Can you work these out from the model? Positions are in its coordinate system, mm. A direction names the side the tool comes from. Give positions to 0.01 mm unless a question says otherwise; leave off trailing zeros. Write each loop counter-clockwise with the first axis right and the second up, starting at its lowest first coordinate (ties: lowest second). Pieces come first, ordered by that corner, then holes. Notation, with made-up numbers: (25.5, -27) -> (69.5, -27) arc R18 cw to (69.5, -6) -> close; hole circle Ø6 at (68.25, -10). An arc over 180 degrees is marked (long way). One line per item, written item: value.
Autodesk Inventor part; units mm, degrees
ref_plane "YZ Plane" through (0, 0, 0) normal (1, 0, 0) x (0, 1, 0)
ref_plane "XZ Plane" through (0, 0, 0) normal (0, 1, 0) x (-1, 0, 0)
ref_plane "XY Plane" through (0, 0, 0) normal (0, 0, 1) x (1, 0, 0)
sketch "Sketch1" plane through (0, 0, 0) normal (0, 1, 0) x (-1, 0, 0)
  line L0 (59.6914, -40.823) -> (-60.3086, -40.823)
  line L1 (-65.3086, -35.823) -> (-65.3086, 34.177)
  line L2 (-60.3086, 39.177) -> (59.6914, 39.177)
  line L3 (64.6914, 34.177) -> (64.6914, -35.823)
  arc A0 (59.6914, -40.823) -> (64.6914, -35.823) centre (59.6914, -35.823) ccw
  arc A1 (-65.3086, -35.823) -> (-60.3086, -40.823) centre (-60.3086, -35.823) ccw
  arc A2 (64.6914, 34.177) -> (59.6914, 39.177) centre (59.6914, 34.177) ccw
  arc A3 (-60.3086, 39.177) -> (-65.3086, 34.177) centre (-60.3086, 34.177) ccw
  point P0 (0, 0)
  point P1 (64.6914, -40.823)
  point P2 (-65.3086, 39.177)
  point P3 (64.6914, 39.177)
  dimension "d0" = 80
  dimension "d1" = 130
  dimension "d2" = 5
  dimension "d3" = 5
  dimension "d4" = 5
  dimension "d5" = 5
extrude "Extrusion1" add sketch "Sketch1" along normal blind 2
sketch "Sketch2" plane through (0, 2, 0) normal (0, 1, 0) x (1, 0, 0)
  line L0 (-64.6914, 35.823) -> (-64.6914, -34.177)
  line L1 (-64.6914, 35.823) -> (-64.6914, -34.177)
  arc A0 (-64.6914, -34.177) -> (-59.6914, -39.177) centre (-59.6914, -34.177) ccw
  arc A1 (-64.6914, -34.177) -> (-59.6914, -39.177) centre (-59.6914, -34.177) ccw
  arc A2 (-59.6914, 40.823) -> (-64.6914, 35.823) centre (-59.6914, 35.823) ccw
  arc A3 (65.3086, 35.823) -> (60.3086, 40.823) centre (60.3086, 35.823) ccw
  arc A4 (65.3086, 35.823) -> (60.3086, 40.823) centre (60.3086, 35.823) ccw
  line L2 (-62.1914, 35.823) -> (-62.1914, -34.177)
  line L3 (65.3086, -34.177) -> (65.3086, 35.823)
  line L4 (65.3086, 35.823) -> (65.3086, -34.177)
  arc A5 (60.3086, -39.177) -> (65.3086, -34.177) centre (60.3086, -34.177) ccw
  line L5 (-59.6914, -39.177) -> (60.3086, -39.177)
  line L6 (60.3086, -39.177) -> (-59.6914, -39.177)
  line L7 (60.3086, 40.823) -> (-59.6914, 40.823)
  line L8 (-59.6914, 40.823) -> (60.3086, 40.823)
  line L9 (62.8086, 35.823) -> (62.8086, -34.177)
  line L10 (60.3086, -36.677) -> (-59.6914, -36.677)
  line L11 (-59.6914, 38.323) -> (60.3086, 38.323)
  arc A6 (-59.6914, 38.323) -> (-62.1914, 35.823) centre (-59.6914, 35.823) ccw
  arc A7 (62.8086, 35.823) -> (60.3086, 38.323) centre (60.3086, 35.823) ccw
  arc A8 (60.3086, -36.677) -> (62.8086, -34.177) centre (60.3086, -34.177) ccw
  arc A9 (-62.1914, -34.177) -> (-59.6914, -36.677) centre (-59.6914, -34.177) ccw
  arc A10 (-59.6914, 39.323) -> (-63.1914, 35.823) centre (-59.6914, 35.823) ccw
  arc A11 (63.8086, 35.823) -> (60.3086, 39.323) centre (60.3086, 35.823) ccw
  arc A12 (60.3086, -37.677) -> (63.8086, -34.177) centre (60.3086, -34.177) ccw
  arc A13 (-63.1914, -34.177) -> (-59.6914, -37.677) centre (-59.6914, -34.177) ccw
  line L12 (-63.1914, 35.823) -> (-63.1914, -34.177)
  line L13 (-59.6914, -37.677) -> (60.3086, -37.677)
  line L14 (63.8086, -34.177) -> (63.8086, 35.823)
  line L15 (60.3086, 39.323) -> (-59.6914, 39.323)
  line L16 (-59.6914, 32.323) -> (-62.1914, 32.323)
  line L17 (-56.1914, 35.823) -> (-56.1914, 38.323)
  arc A14 (-59.6914, 32.323) -> (-56.1914, 35.823) centre (-59.6914, 35.823) ccw
  line L18 (0.3086, 40.823) -> (0.3086, 33.323)
  line L19 (65.3086, 0.823) -> (44.6486, 0.823)
  line L20 (60.3086, 32.323) -> (62.8086, 32.323)
  line L21 (56.8086, 35.823) -> (56.8086, 38.323)
  arc A15 (56.8086, 35.823) -> (60.3086, 32.323) centre (60.3086, 35.823) ccw
  line L22 (-59.6914, -30.677) -> (-62.1914, -30.677)
  line L23 (-56.1914, -34.177) -> (-56.1914, -36.677)
  arc A16 (-56.1914, -34.177) -> (-59.6914, -30.677) centre (-59.6914, -34.177) ccw
  line L24 (56.8086, -34.177) -> (56.8086, -36.677)
  arc A17 (60.3086, -30.677) -> (56.8086, -34.177) centre (60.3086, -34.177) ccw
  line L25 (60.3086, -30.677) -> (62.8086, -30.677)
  point P0 (0, 0)
  point P1 (60.3086, -34.2192)
  point P2 (65.3086, -34.2192)
  point P3 (59.6599, -39.177)
  point P4 (56.8086, 38.323)
  point P5 (62.8086, -30.677)
  point P6 (56.8086, -36.677)
  point P7 (-56.1914, -36.677)
  point P8 (-62.1914, -30.677)
  dimension "d51" = 5
  dimension "d8" = 2.5
  dimension "d9" = 2.5
  dimension "d10" = 2.5
  dimension "d11" = 2.5
  dimension "d12" = 7
  dimension "d13" = 7
  dimension "d14" = 7
  dimension "d15" = 7
  dimension "d34" = 3.5
  dimension "d50" = 2.5
  dimension "d52" = 5
  dimension "d53" = 2.5
extrude "Extrusion2" add sketch "Sketch2" along normal blind 5 contours A2 L7 L18 L15 A10 L12 A13 L13 A12 L14 L19 L3 A5 L5 A0 L0 | L7 A3 L3 L19 L14 A11 L15 L18 | L17 A14 L16 L2 A6 L11 | L11 A7 L9 L20 A15 L21 | L9 A8 L10 L24 A17 L25 | L22 A16 L23 L10 A9 L2
extrude "Extrusion3" add sketch "Sketch2" along normal blind 6 contours L18 L11 A6 L2 A9 L10 A8 L9 L19 L14 A12 L13 A13 L12 A10 L15 | L15 A11 L14 L19 L9 A7 L11 L18 | L17 A14 L16 L2 A6 L11 | L11 A7 L9 L20 A15 L21 | L9 A8 L10 L24 A17 L25 | L22 A16 L23 L10 A9 L2
sketch "Sketch3" plane through (0, 0, 0) normal (0, -1, 0) x (1, 0, 0)
  circle A0 centre (60.3086, 34.177) radius 3
  line L0 (-59.6914, 39.177) -> (60.3086, 39.177)
  line L1 (65.3086, 34.177) -> (65.3086, -35.823)
  line L2 (65.3086, 24.0261) -> (65.3086, 17.2129)
  line L3 (38.477, 39.177) -> (29.3328, 39.177)
  line L4 (-59.6914, 39.177) -> (60.3086, 39.177)
  circle A1 centre (60.3086, -35.823) radius 3
  circle A2 centre (-59.6914, 34.177) radius 3
  circle A3 centre (-59.6914, -35.823) radius 3
  line L5 (-64.6914, -35.823) -> (-64.6914, 34.177)
  line L6 (60.3086, -40.823) -> (-59.6914, -40.823)
  point P0 (0, 0)
  point P1 (33.602, 39.1426)
  point P2 (55.3086, 34.177)
  point P3 (65.3086, -35.823)
  dimension "d20" = 6
  dimension "d21" = 5
  dimension "d26" = 70
  dimension "d29" = 120
  dimension "d54" = 130
  dimension "d55" = 80
  dimension "d56" = 5
extrude "Extrusion4" cut sketch "Sketch3" against normal blind 3
sketch "Sketch4" plane through (60.3086, 3, -35.823) normal (0, -1, 0) x (1, 0, 0)
  circle A0 centre (0, 0) radius 3
  point P0 (-60.3086, 35.823)
hole "Hole1" at (60.3086, 3, -35.823) direction (0, 1, 0) diameter 3.5 end through all
pattern_linear "Rectangular Pattern1" count 2 spacing 120 along (-1, 0, 0) count 2 spacing 70 along (0, 0, 1) of "Hole1"
chamfer "Chamfer1" distance 1 angle 45 8 edges at (0.3086, 0, 39.177) (63.8442, 0, 37.7125) (65.3086, 0, -0.823) (63.8442, 0, -39.3586) (0.3086, 0, -40.823) (-63.2269, 0, -39.3586) (-64.6914, 0, -0.823) (-63.2269, 0, 37.7125)
sketch "Sketch9" plane through (0, 0, 0) normal (0, -1, 0) x (1, 0, 0)
  line L0 (-8.8254, 34.5739) -> (9.2353, 34.5739) construction
  line L1 (9.2353, 34.5739) -> (9.2353, 29.7737) construction
  line L2 (9.2353, 29.7737) -> (-8.8254, 29.7737) construction
  line L3 (-8.8254, 29.7737) -> (-8.8254, 34.5739) construction
  point P0 (0, 0)
sketch "Sketch10" plane through (0, 2, 0) normal (0, 1, 0) x (1, 0, 0)
  line L0 (46.8086, -34.677) -> (-3.1914, -34.677)
  line L1 (-3.1914, -34.677) -> (-3.1914, -32.677)
  line L2 (-3.1914, -32.677) -> (46.8086, -32.677)
  line L3 (46.8086, -32.677) -> (46.8086, -34.677)
  line L4 (56.8086, -34.177) -> (56.8086, -36.677)
  line L5 (56.8086, -36.677) -> (-56.1914, -36.677)
  line L6 (-46.1914, 36.323) -> (3.8086, 36.323)
  line L7 (3.8086, 36.323) -> (3.8086, 34.323)
  line L8 (3.8086, 34.323) -> (-46.1914, 34.323)
  line L9 (-46.1914, 34.323) -> (-46.1914, 36.323)
  line L10 (-56.1914, 38.323) -> (56.8086, 38.323)
  line L11 (-56.1914, 35.823) -> (-56.1914, 38.323)
  point P0 (0, 0)
  point P1 (56.8086, -35.427)
  point P2 (46.8086, -33.677)
  point P3 (-3.1914, -36.677)
  point P4 (-46.1914, 35.323)
  point P5 (-56.1914, 37.073)
  dimension "d97" = 50
  dimension "d98" = 2
  dimension "d99" = 10
  dimension "d100" = 2
  dimension "d110" = 50
  dimension "d111" = 2
  dimension "d112" = 2
  dimension "d113" = 10
extrude "Extrusion7" add sketch "Sketch10" along normal blind 5
chamfer "Chamfer2" distance 1 angle 60 1 edges at (21.8086, 7, 34.677) measured on face at (13.4753, 7, 33.3436)
chamfer "Chamfer4" distance 1 angle 60 1 edges at (-21.1914, 7, -36.323) measured on face at (-29.5247, 7, -35.6564)
sketch "Sketch11" plane through (0, 0, 0) normal (0, -1, 0) x (1, 0, 0)
  line L0 (-56.6914, 5.177) -> (-16.6914, 5.177)
  line L1 (-16.6914, 5.177) -> (-16.6914, -20.823)
  line L2 (-16.6914, -20.823) -> (-56.6914, -20.823)
  line L3 (-56.6914, -20.823) -> (-56.6914, 5.177)
  line L4 (-64.6914, 34.177) -> (-64.6914, -35.823)
  line L5 (-59.6914, -40.823) -> (60.3086, -40.823)
  point P0 (0, 0)
  dimension "d117" = 40
  dimension "d118" = 26
  dimension "d119" = 8
  dimension "d120" = 20
extrude "Extrusion8" cut sketch "Sketch11" against normal blind 10
sketch "Sketch12" plane through (0, 2, 0) normal (0, 1, 0) x (1, 0, 0)
  line L0 (-57.6914, 28.823) -> (-15.6914, 28.823)
  line L1 (-15.6914, 28.823) -> (-15.6914, -13.177)
  line L2 (-15.6914, -13.177) -> (-57.6914, -13.177)
  line L3 (-57.6914, -13.177) -> (-57.6914, 28.823)
  line L4 (-16.6914, -5.177) -> (-56.6914, -5.177)
  line L5 (-16.6914, 20.823) -> (-16.6914, -5.177)
  circle A0 centre (-54.1914, 25.323) radius 1.75
  circle A1 centre (-19.1914, 25.323) radius 1.75
  circle A2 centre (-54.1914, -9.677) radius 1.75
  circle A3 centre (-19.1914, -9.677) radius 1.75
  point P0 (0, 0)
  dimension "d127" = 42
  dimension "d128" = 42
  dimension "d129" = 8
  dimension "d130" = 1
  dimension "d131" = 3.5
  dimension "d132" = 3.5
  dimension "d133" = 3.5
  dimension "d136" = 35
  dimension "d139" = 35
extrude "Extrusion9" cut sketch "Sketch12" against normal blind 10 contours A0 | A1 | A2 | A3
sketch "Sketch13" plane through (0, 2, 0) normal (0, 1, 0) x (1, 0, 0)
  line L0 (-57.6914, -6.177) -> (-15.6914, -6.177)
  line L1 (-15.6914, -6.177) -> (-15.6914, 21.823)
  line L2 (-15.6914, 21.823) -> (-57.6914, 21.823)
  line L3 (-57.6914, 21.823) -> (-57.6914, -6.177)
  line L4 (-56.6914, 20.823) -> (-16.6914, 20.823)
  line L5 (-56.6914, -5.177) -> (-16.6914, -5.177)
  line L6 (-16.6914, -5.177) -> (-16.6914, 20.823)
  line L7 (-16.6914, 20.823) -> (-56.6914, 20.823)
  line L8 (-56.6914, 20.823) -> (-56.6914, -5.177)
  point P0 (0, 0)
  dimension "d144" = 1
  dimension "d145" = 1
  dimension "d146" = 1
  dimension "d147" = 1
extrude "Extrusion10" add sketch "Sketch13" along normal blind 3.8
equation "\"d3\" = d2"
equation "\"d4\" = d2"
equation "\"d5\" = d2"
equation "\"d9\" = d8"
equation "\"d10\" = d8"
equation "\"d11\" = d8"
equation "\"d52\" = d51"
equation "\"d53\" = d50"
properties part number "housing_top"
1) If we section it at D-D (x = 38): Write out the boundary of the cut face in (y, z), and give its area (3 significant figures).
Answer list:
outline: (0, -39.82) -> (1, -40.82) -> (7, -40.82) -> (7, -39.32) -> (8, -39.32) -> (8, -38.32) -> (2, -38.32) -> (2, 32.68) -> (7, 32.68) -> (7, 33.68) -> (5.27, 34.68) -> (2, 34.68) -> (2, 36.68) -> (8, 36.68) -> (8, 37.68) -> (7, 37.68) -> (7, 39.18) -> (1, 39.18) -> (0, 38.18) -> close
area: 195 mm^2
2) Will these pins go through, and if not, where does the flat tip stop? pin 1 (22.5 mm diameter, centred on x = -1.5, z = -7, fed in from +Y); pin 2 (14 mm diameter, centred on x = -32, z = -12.5, fed in from +Y); pin 3 (0.8 mm diameter, centred on y = 7.5, z = -10, fed in from +X); pin 4 (1.1 mm diameter, centred on x = -25, z = -35, fed in from +Y).
Answer list:
pin 1: stops at y = 2
pin 2: passes through
pin 3: stops at x = 63.81
pin 4: stops at y = 7
3) I need wall thicknesses on L1, parallel to Z at x = 41.5, y = 4; L2, parallel to Z at x = 60.5, y = 5; L3, parallel to X at y = 4.5, z = -13. Which ranges of each line are inside material? Lowest first, please.
Answer list:
L1: z = -40.82 to -38.32, 32.68 to 34.68, 36.68 to 39.18
L2: z = -40.82 to -37.56, -34.08 to -32.32, 30.68 to 32.44, 35.92 to 39.17
L3: x = -64.69 to -62.19, -57.69 to -56.69, -16.69 to -15.69, 62.81 to 65.31
4) If we section it at C-C (x = -37): Write out the boundary of the cut face in (y, z).
Answer list:
outline: (0, -39.82) -> (1, -40.82) -> (7, -40.82) -> (7, -39.32) -> (8, -39.32) -> (8, -38.32) -> (2, -38.32) -> (2, -36.32) -> (5.27, -36.32) -> (7, -35.32) -> (7, -34.32) -> (2, -34.32) -> (2, -21.82) -> (5.8, -21.82) -> (5.8, -20.82) -> (0, -20.82) -> close; (0, 5.18) -> (5.8, 5.18) -> (5.8, 6.18) -> (2, 6.18) -> (2, 36.68) -> (8, 36.68) -> (8, 37.68) -> (7, 37.68) -> (7, 39.18) -> (1, 39.18) -> (0, 38.18) -> close
5) If we section it at B-B (z = -7): Write out the boundary of the cut face in (x, y), and give its area (3 significant figures).
Answer list:
outline: (-64.69, 1) -> (-63.69, 0) -> (-56.69, 0) -> (-56.69, 5.8) -> (-57.69, 5.8) -> (-57.69, 2) -> (-62.19, 2) -> (-62.19, 8) -> (-63.19, 8) -> (-63.19, 7) -> (-64.69, 7) -> close; (-16.69, 0) -> (64.31, 0) -> (65.31, 1) -> (65.31, 7) -> (63.81, 7) -> (63.81, 8) -> (62.81, 8) -> (62.81, 2) -> (-15.69, 2) -> (-15.69, 5.8) -> (-16.69, 5.8) -> close
area: 214 mm^2
6) If we section it at A-A (x = -50): Write out the boundary of the cut face in (y, z).
Answer list:
outline: (0, -39.82) -> (1, -40.82) -> (7, -40.82) -> (7, -39.32) -> (8, -39.32) -> (8, -38.32) -> (2, -38.32) -> (2, -21.82) -> (5.8, -21.82) -> (5.8, -20.82) -> (0, -20.82) -> close; (0, 5.18) -> (5.8, 5.18) -> (5.8, 6.18) -> (2, 6.18) -> (2, 36.68) -> (8, 36.68) -> (8, 37.68) -> (7, 37.68) -> (7, 39.18) -> (1, 39.18) -> (0, 38.18) -> close
7) For faces 4 (the face through (-37, 4, 6.177)), 5 (the face through (62, 3, 33)), 6 (the face through (62.811, 7.493, 36.625)), which set-ups out of +Z, -Z, +X, -X, +Y, -Y let a thin tool reach every point of the face, with its end or its side?
Answer list:
face 4: +Y
face 5: -Y
face 6: +Z, +X, +Y
8) We'd pull the mould along Z, two halves only. Please class faces 1 (the face through (63.883, 3.958, 37.673)), 2 (the face through (-1, 4, -40.823)), 3 (the face through (-55.58, 1.01, -24.26)): released by +Z, released by -Z, zero draft, split by the parting line, or undercut.
Answer list:
face 1: released by +Z
face 2: released by -Z
face 3: undercut
